Read the model definition and answer for the solid it produces. Units are mm, in the model's axes. A direction names the side the tool comes from. Coordinates: 2 decimals unless noted, no trailing zeros. Order: outer loops, then holes, each group sorted by start corner. A loop starts at its lowest first (then second) coordinate and runs counter-clockwise, first axis right, second up. Notation, with made-up numbers: M -16.5,24.25 L 0.5,24.25 A18 cw 0.5,34.25 Z; hole C -20,85 d4. An arc over 180 degrees is marked long. Use a Markdown table: item, result. Add a question column.
1) For faces 1 (the face through (72.956, 72.708, -25.092)), 2 (the face through (71.645, 71.397, -11.094)), 3 (the face through (67.425, 80.148, -5.324)), 4 (the face through (72.658, 85.239, -5.324)), 5 (the face through (74.582, 80.698, -5.324)), determine the directions among +Z, -Z, +X, -X, +Y, -Y from which every point of the face is accessible in a straight line to the end or side of a thin tool.
2) Each of these flat-tipped pins is pushed along its axis until it touches: pin 1 Ø2 at (y, z) = (77.5, -21) entering from +X; pin 2 Ø1 at (x, z) = (72, -12) entering from -Y; pin 3 Ø3 at (x, z) = (72, -10.5) entering from -Y; pin 4 Ø3 at (x, y) = (81.5, 71.5) entering from -Z. Where does it stop, or does it pass through?
3) The mould has two halves that part along Y. Classify faces 6 (the face through (69, 83, -3.6)), 7 (the face through (72.25, 72, -6.01)), 8 (the face through (83.01, 72.81, -19.17)), 9 (the face through (80.73, 80.49, -13.5)): released by +Y, released by -Y, zero draft, split by the parting line, or undercut.
4) Find section A-A on z = -11.5. Write down the section's boundary in (x, y), plus the area to 3 significant figures.
5) Find section B-B on z = 2. Write down the section's boundary in (x, y), plus the area to 3 significant figures.
6) Find the intervals of material crossed by probe 1 along X at (y, z) = (69.75, -11.5); probe 2 along Y at (x, z) = (70.25, 2.5); probe 3 along Z at (x, y) = (70.75, 85.5), in increasing order. Write a range as [from, to].
from build123d import *

# Parameters (mm, degrees)
PAD022_DEPTH            = 12.5
SKETCH043_R             = 2.2
POCKET007_DEPTH         = 35.501
POCKET098_DEPTH         = 3.4
BODY022_PLACEMENT_ANGLE = 45


with BuildPart() as part:
    # Sketch042 → Pad022 (new body, symmetric)
    with BuildSketch(Plane.YZ):
        with BuildLine():
            Line((-1, 28.5), (-1, 21.385113))
            Line((-1, 21.385113), (-2.732051, 18.385113))
            ThreePointArc((-2.732051, 18.385113), (-3, 17.385113), (-2.732051, 16.385113))
            Line((-2.732051, 16.385113), (0, 11.653062))
            Line((0, 11.653062), (0, 0))
            Line((0, 0), (11, 0))
            Line((11, 0), (11, 35.5))
            Line((11, 35.5), (-8, 35.5))
            Line((-8, 35.5), (-8, 31.5))
            Line((-8, 31.5), (-2.5, 31.5))
            add(Edge.make_bspline(
                [(-1, 28.5), (-1, 31.5), (-2.5, 31.5)],
                knots=[4.712389, 4.712389, 4.712389, 6.283185, 6.283185, 6.283185], degree=2, weights=[1, 0.707107, 1]))
        make_face()
    extrude(amount=PAD022_DEPTH, both=True)

    # Sketch043 → Pocket007 (cut, through all)
    with BuildSketch(Plane.XY):
        with Locations((-7.5, 5)):
            Circle(SKETCH043_R)
        with Locations((7.5, 5)):
            Circle(SKETCH043_R)
        with BuildLine():
            ThreePointArc((-12.5, -3.784326), (0, -8), (12.5, -3.784326))
            Line((12.5, -3.784326), (13.5, -3.784326))
            Line((13.5, -3.784326), (13.5, -9))
            Line((-13.5, -9), (13.5, -9))
            Line((-13.5, -3.784326), (-13.5, -9))
            Line((-12.5, -3.784326), (-13.5, -3.784326))
        make_face()
    extrude(amount=POCKET007_DEPTH, mode=Mode.SUBTRACT)

    # Sketch150 → Pocket098 (cut)
    with BuildSketch(Plane.XY.offset(24)):
        Polygon((-5.392672, 1.35), (-3.285343, 5), (-5.392672, 8.65), (-13.5, 8.65), (-13.5, 1.35), align=None)
        Polygon((5.392672, 8.65), (3.285343, 5), (5.392672, 1.35), (13.5, 1.35), (13.5, 8.65), align=None)
    extrude(amount=POCKET098_DEPTH, mode=Mode.SUBTRACT)


with BuildPart() as part_1:
    # Body022 placement: moved
    add(part.part.moved(Location((72.831998, 72.831998, -31))).rotate(Axis((72.831998, 72.831998, -31), (0, 0, -1)), BODY022_PLACEMENT_ANGLE))


solid = part_1.part
Check result:
| question | item | result |
|---|---|---|
| 1 | face 1 | -Z, -X, -Y |
| 1 | face 2 | -X, -Y |
| 1 | face 3 | +Y |
| 1 | face 4 | -X |
| 1 | face 5 | none |
| 2 | pin 1 | stops at x = 84.72 |
| 2 | pin 2 | stops at y = 69.66 |
| 2 | pin 3 | stops at y = 69.59 |
| 2 | pin 4 | passes through |
| 3 | face 6 | undercut |
| 3 | face 7 | released by -Y |
| 3 | face 8 | undercut |
| 3 | face 9 | released by +Y |
| 4 | outline | M 62.52,80.19 L 80.19,62.52 L 89.45,71.77 L 71.77,89.45 Z; hole C 71.06,81.67 d4.4; hole C 81.67,71.06 d4.4 |
| 4 | area | 297 mm2 |
| 5 | outline | M 61.32,78.99 A20.64 ccw 78.99,61.32 L 89.45,71.77 L 71.77,89.45 Z; hole C 71.06,81.67 d4.4; hole C 81.67,71.06 d4.4 |
| 5 | area | 411 mm2 |
| 6 | probe 1 | x = [72.96, 79.91], [83.44, 87.43] |
| 6 | probe 2 | y = [64.64, 79.63], [83.71, 87.93] |
| 6 | probe 3 | z = [-31, -7], [-3.6, 4.5] |
